Autodesk Inventor part; units mm, degrees
ref_plane "YZ Plane" through (0, 0, 0) normal (1, 0, 0) x (0, 1, 0)
ref_plane "XZ Plane" through (0, 0, 0) normal (0, 1, 0) x (-1, 0, 0)
ref_plane "XY Plane" through (0, 0, 0) normal (0, 0, 1) x (1, 0, 0)
sketch "Esboço1" plane through (0, 0, 0) normal (0, 1, 0) x (-1, 0, 0)
  line L0 (0, 0) -> (80, 0)
  line L1 (80, 0) -> (80, -80)
  line L2 (80, -80) -> (0, -80)
  line L3 (0, -80) -> (0, 0)
  circle A0 centre (40, -40) radius 5
  dimension "d0" = 80
  dimension "d1" = 80
  dimension "d2" = 10
extrude "Extrusão1" add sketch "Esboço1" along normal blind 12
fillet "Arredondamento1" radius 10 4 edges at (-80, 6, 0) (0, 6, 0) (0, 6, -80) (-80, 6, -80)
sketch "Esboço2" plane through (0, 12, 0) normal (0, 1, 0) x (1, 0, 0)
  point P0 (0, 0)
properties part number "Corpo_1"
For this review, take the finished solid that the model builds, in its own axes (mm). Coordinates: 2 decimals unless noted, no trailing zeros. Loops run counter-clockwise (first coordinate to the right, second up) from the corner with the lowest first, then second, coordinate; pieces in that order, holes last.
1. Add section A-A, the plane x = -40. Give the boundary of the cut face in (y, z), then the cut area to 3 significant figures.
2. Add section C-C, the plane y = 8. Give the boundary of the cut face in (x, z).
3. Add section B-B, the plane z = -40. Give the boundary of the cut face in (x, y).
4. Insertion check: P1, Ø8, axis at x = -40, z = -40, coming from the +Y side. The pin has a flat end and moves straight along its axis. Give the tip position at first contact, or say it passes through.
5. For line 1 (Z direction, x = -40, y = 4.75); line 2 (Z direction, x = -36, y = 9.5); line 3 (X direction, y = 10.5, z = -6.5), list the stretches that pass through material, from the lowest coordinate up.
6. Mouldability with a two-part tool opening along Z and no side actions: class faces 1 (the cylindrical face through (-76.99, 6.08, -77.15)), 2 (the cylindrical face through (-77.15, 6.08, -3.01)), 3 (the flat face through (-48, 0, -39)), 4 (the cylindrical face through (-36, 6, -43)) as +Z half, -Z half, draft (parallel to the pull), parting line (faces both ways), or undercut.
7. Add section D-D, the plane x = -73.5. Give the boundary of the cut face in (y, z), then the cut area to 3 significant figures.
Result:
1. outline: (0, -80) - (12, -80) - (12, -45) - (0, -45) - close; (0, -35) - (12, -35) - (12, 0) - (0, 0) - close
1. area: 840 mm2
2. outline: (-80, -70) arc R10 ccw to (-70, -80) - (-10, -80) arc R10 ccw to (0, -70) - (0, -10) arc R10 ccw to (-10, 0) - (-70, 0) arc R10 ccw to (-80, -10) - close; hole circle Ø10 at (-40, -40)
3. outline: (-80, 0) - (-45, 0) - (-45, 12) - (-80, 12) - close; (-35, 0) - (0, 0) - (0, 12) - (-35, 12) - close
4. P1: passes through
5. line 1: z = -80 to -45, -35 to 0
5. line 2: z = -80 to -43, -37 to 0
5. line 3: x = -79.37 to -0.63
6. face 1: -Z half
6. face 2: +Z half
6. face 3: draft
6. face 4: undercut
7. outline: (0, -79.37) - (12, -79.37) - (12, -0.63) - (0, -0.63) - close
7. area: 945 mm2
